```python
from build123d import *

# Parameters (mm, degrees)
BOSS_EXTRUDE2_DEPTH      = 3.5
CUT_EXTRUDE3_DEPTH       = 161.765145163
CUT_EXTRUDE3_DEPTH_BACK  = 161.765145163
SKETCH3_R                = 1.625
CUT_EXTRUDE6_DEPTH       = 161.765145163
CUT_EXTRUDE6_DEPTH_BACK  = 161.765145163
SKETCH6_R                = 15
SKETCH8_R                = 1.5
CUT_EXTRUDE7_DEPTH       = 3.5
CIRPATTERN1_COUNT        = 4
CUT_EXTRUDE12_DEPTH      = 161.765145163
CUT_EXTRUDE12_DEPTH_BACK = 161.765145163
SKETCH20_W               = 15
SKETCH20_H               = 15
FILLET2_R                = 25
FILLET3_R                = 4
SKETCH21_R               = 2.5
BOSS_EXTRUDE4_DEPTH      = 3
SKETCH22_R               = 1.6
CUT_EXTRUDE13_DEPTH      = 158.947840775
SKETCH24_R               = 2.4
BOSS_EXTRUDE6_DEPTH      = 3.5
CUT_EXTRUDE14_DEPTH      = 158.969207144
CUT_EXTRUDE14_DEPTH_BACK = 158.969207144
SKETCH25_R               = 1.6
CUT_EXTRUDE15_DEPTH      = 158.852844148
CUT_EXTRUDE15_DEPTH_BACK = 158.852844148
SKETCH26_R               = 9.404630818
CUT_EXTRUDE16_DEPTH      = 158.852844148
CUT_EXTRUDE16_DEPTH_BACK = 158.852844148
CUT_EXTRUDE17_DEPTH      = 158.969207144
CUT_EXTRUDE17_DEPTH_BACK = 158.969207144
SKETCH28_R               = 10


with BuildPart() as part:
    # Sketch1 → Boss-Extrude2 (new body)
    with BuildSketch(Plane(origin=(0, 0, 0), x_dir=(1, 0, 0), z_dir=(0, 1, 0))):
        Polygon((0, -113.651181031), (80.363520797, -80.363520797), (113.651181031, 0), (80.363520797, 80.363520797), (0, 113.651181031), (-80.363520797, 80.363520797), (-113.651181031, 0), (-80.363520797, -80.363520797), align=None)
    extrude(amount=BOSS_EXTRUDE2_DEPTH)

    # Sketch3 → Cut-Extrude3 (cut, two sides: drawn at the far end of the back side and taken through both)
    with BuildSketch(Plane(origin=(0, 3.5, 0), x_dir=(1, 0, 0), z_dir=(0, 1, 0)).offset(-CUT_EXTRUDE3_DEPTH_BACK)):
        with Locations(Location((-75, -75, 0), (0, 0, 270))):
            Circle(SKETCH3_R)
        with Locations(Location((75, -75, 0), (0, 0, 270))):
            Circle(SKETCH3_R)
        with Locations(Location((75, 75, 0), (0, 0, 270))):
            Circle(SKETCH3_R)
        with Locations(Location((-75, 75, 0), (0, 0, 270))):
            Circle(SKETCH3_R)
    extrude(amount=CUT_EXTRUDE3_DEPTH + CUT_EXTRUDE3_DEPTH_BACK, mode=Mode.SUBTRACT)

    # Sketch6 → Cut-Extrude6 (cut, two sides: drawn at the far end of the back side and taken through both)
    with BuildSketch(Plane(origin=(0, 3.5, 0), x_dir=(1, 0, 0), z_dir=(0, 1, 0)).offset(-CUT_EXTRUDE6_DEPTH_BACK)):
        with Locations(Location((0, 0, 0), (0, 0, 270))):
            Circle(SKETCH6_R)
    extrude(amount=CUT_EXTRUDE6_DEPTH + CUT_EXTRUDE6_DEPTH_BACK, mode=Mode.SUBTRACT)

    # Sketch8 → Cut-Extrude7 (cut)
    with BuildSketch(Plane(origin=(0, 3.5, 0), x_dir=(1, 0, 0), z_dir=(0, 1, 0))):
        with Locations(Location((-15, -71.401181031, 0), (0, 0, 270))):
            Circle(SKETCH8_R)
        with Locations(Location((15, -71.401181031, 0), (0, 0, 270))):
            Circle(SKETCH8_R)
        with Locations(Location((-15, -101.151181031, 0), (0, 0, 270))):
            Circle(SKETCH8_R)
        with Locations(Location((15, -101.151181031, 0), (0, 0, 270))):
            Circle(SKETCH8_R)
    cut_extrude7 = extrude(amount=-CUT_EXTRUDE7_DEPTH, mode=Mode.SUBTRACT)

    # CirPattern1: Cut-Extrude7 ×4 about axis
    cirpattern1_axis = Axis((0, 0, 0), (0, 1, 0))
    for i in range(1, CIRPATTERN1_COUNT):
        add(cut_extrude7.rotate(cirpattern1_axis, i * 360 / CIRPATTERN1_COUNT), mode=Mode.SUBTRACT)

    # Sketch20 → Cut-Extrude12 (cut, two sides: drawn at the far end of the back side and taken through both)
    with BuildSketch(Plane(origin=(0, 3.5, 0), x_dir=(1, 0, 0), z_dir=(0, 1, 0)).offset(-CUT_EXTRUDE12_DEPTH_BACK)):
        with Locations((33.5, 78.901181031)):
            Rectangle(SKETCH20_W, SKETCH20_H)
    extrude(amount=CUT_EXTRUDE12_DEPTH + CUT_EXTRUDE12_DEPTH_BACK, mode=Mode.SUBTRACT)

    # Fillet2
    fillet2_edges = [part.edges().sort_by_distance(p)[0] for p in [
        (-113.651181031, 1.75, 0),
        (0, 1.75, -113.651181031),
        (113.651181031, 1.75, 0),
        (0, 1.75, 113.651181031),
    ]]
    fillet(fillet2_edges, radius=FILLET2_R)

    # Fillet3
    fillet3_edges = [part.edges().sort_by_distance(p)[0] for p in [
        (41, 1.75, -86.401181031),
    ]]
    fillet(fillet3_edges, radius=FILLET3_R)

    # Sketch21 → Boss-Extrude4 (add)
    with BuildSketch(Plane.XZ):
        with Locations(Location((-8.867969273, 25.52523978, 0), (0, 0, 90))):
            Circle(SKETCH21_R)
        with Locations(Location((25.310885524, -8.653615016, 0), (0, 0, 90))):
            Circle(SKETCH21_R)
        with Locations(Location((44.25922594, 78.652434993, 0), (0, 0, 90))):
            Circle(SKETCH21_R)
        with Locations(Location((83.736431848, 49.771931307, 0), (0, 0, 90))):
            Circle(SKETCH21_R)
    extrude(amount=BOSS_EXTRUDE4_DEPTH)

    # Sketch22 → Cut-Extrude13 (cut, through all)
    with BuildSketch(Plane.XZ.offset(3)):
        with Locations(Location((83.736431848, 49.771931307, 0), (0, 0, 270))):
            Circle(SKETCH22_R)
        with Locations(Location((25.310885524, -8.653615016, 0), (0, 0, 270))):
            Circle(SKETCH22_R)
        with Locations(Location((-8.867969273, 25.52523978, 0), (0, 0, 270))):
            Circle(SKETCH22_R)
        with Locations(Location((44.25922594, 78.652434993, 0), (0, 0, 270))):
            Circle(SKETCH22_R)
    extrude(amount=-CUT_EXTRUDE13_DEPTH, mode=Mode.SUBTRACT)

    # Sketch24 → Boss-Extrude6 (add)
    with BuildSketch(Plane.XZ):
        with Locations(Location((-64.472580457, -31.0267951, 0), (0, 0, 90))):
            Circle(SKETCH24_R)
        with Locations(Location((-29.019501349, -37.278129496, 0), (0, 0, 90))):
            Circle(SKETCH24_R)
        with Locations(Location((-35.270835745, -72.731208605, 0), (0, 0, 90))):
            Circle(SKETCH24_R)
        with Locations(Location((-70.723914853, -66.479874209, 0), (0, 0, 90))):
            Circle(SKETCH24_R)
    extrude(amount=BOSS_EXTRUDE6_DEPTH)

    # Sketch25 → Cut-Extrude14 (cut, two sides: drawn at the far end of the back side and taken through both)
    with BuildSketch(Plane.XZ.offset(3.5).offset(-CUT_EXTRUDE14_DEPTH_BACK)):
        with Locations(Location((-29.019501349, -37.278129496, 0), (0, 0, 270))):
            Circle(SKETCH25_R)
        with Locations(Location((-64.472580457, -31.0267951, 0), (0, 0, 270))):
            Circle(SKETCH25_R)
        with Locations(Location((-70.723914853, -66.479874209, 0), (0, 0, 270))):
            Circle(SKETCH25_R)
        with Locations(Location((-35.270835745, -72.731208605, 0), (0, 0, 270))):
            Circle(SKETCH25_R)
    extrude(amount=CUT_EXTRUDE14_DEPTH + CUT_EXTRUDE14_DEPTH_BACK, mode=Mode.SUBTRACT)

    # Sketch26 → Cut-Extrude15 (cut, two sides: drawn at the far end of the back side and taken through both)
    with BuildSketch(Plane.XZ.offset(-CUT_EXTRUDE15_DEPTH_BACK)):
        with Locations(Location((-60.741403737, 60.741403737, 0), (0, 0, 270))):
            Circle(SKETCH26_R)
        with Locations(Location((60.741403737, -60.741403737, 0), (0, 0, 270))):
            Circle(SKETCH26_R)
    extrude(amount=CUT_EXTRUDE15_DEPTH + CUT_EXTRUDE15_DEPTH_BACK, mode=Mode.SUBTRACT)

    # Sketch27 → Cut-Extrude16 (cut, two sides: drawn at the far end of the back side and taken through both)
    with BuildSketch(Plane.XZ.offset(-CUT_EXTRUDE16_DEPTH_BACK)):
        Polygon((7.39951467, 57.553878611), (11.642155357, 53.311237924), (-9.571048078, 32.098034488), (-13.813688765, 36.340675176), align=None)
        Polygon((32.098034488, -9.571048078), (36.340675176, -13.813688765), (57.553878611, 7.39951467), (53.311237924, 11.642155357), align=None)
    extrude(amount=CUT_EXTRUDE16_DEPTH + CUT_EXTRUDE16_DEPTH_BACK, mode=Mode.SUBTRACT)

    # Sketch28 → Cut-Extrude17 (cut, two sides: drawn at the far end of the back side and taken through both)
    with BuildSketch(Plane(origin=(0, 3.5, 0), x_dir=(1, 0, 0), z_dir=(0, 1, 0)).offset(-CUT_EXTRUDE17_DEPTH_BACK)):
        with Locations(Location((-34.694923367, -27.917780902, 0), (0, 0, 270))):
            Circle(SKETCH28_R)
    extrude(amount=CUT_EXTRUDE17_DEPTH + CUT_EXTRUDE17_DEPTH_BACK, mode=Mode.SUBTRACT)


solid = part.part
```
CAD build for the part. Positions are in the model's coordinates, mm. A direction names the side the tool comes from. Round coordinates to 2 decimals unless told otherwise and drop trailing zeros. Write each loop counter-clockwise with the first axis right and the second up, starting at its lowest first coordinate (ties: lowest second). Pieces come first, ordered by that corner, then holes. Notation, with made-up numbers: (3.5, -10) - (18.5, -10) arc R20 cw to (18.5, 23) - close; hole circle Ø1 at (34.25, 46.25). An arc over 180 degrees is marked (long way). Return JSON: item names as keys, results as strings. Group by question number.
Item 1: Flat gauge pins, fed straight in: pin 1 Ø3 at (y, z) = (1.5, -82.5) entering from +X; pin 2 Ø1 at (y, z) = (0.5, 40) entering from -X; pin 3 Ø2 at (y, z) = (0.5, 43) entering from -X; pin 4 Ø2.5 at (x, z) = (-101.15, -15) entering from -Y. Where does each tip first touch, or does it go through?
Item 2: Band-saw the part on D-D on z = -89. List the corners of the cut face in (x, y), plus the area to 3 significant figures.
Item 3: Mould opens along Z. For faces 1 (the face through (-45.46, 1.73, 94.82)), 2 (the face through (-3.356, 1.774, 46.799)), 3 (the face through (-10.558, -1.479, 23.683)) say: +Z half, -Z half, draft (parallel to the pull), parting line (faces both ways), or undercut.
Item 4: Band-saw the part on A-A on z = 60.5. List the corners of the cut face in (x, y).
Item 5: Band-saw the part on C-C on z = -48. List the corners of the cut face in (x, y), plus the area to 3 significant figures.
Item 6: Band-saw the part on B-B on x = -55.5. List the corners of the cut face in (y, z).
Item 7: 3-axis set-ups, long thin cutter, end or side, ignore diameter. For faces 4 (the face through (-33.142, -1.726, -71.624)), 5 (the face through (46.799, 1.774, -3.356)), 6 (the face through (95.23, 1.73, -44.47)): which of +Z, -Z, +X, -X, +Y, -Y reach the whole face in a straight line?
Item 8: Probe probe 1 along Z at (x, y) = (75, 1.25) (3 decimals); probe 2 along X at (y, z) = (1.75, 0). List the from-to ranges inside material, lowest first.
Resolved:
{
 "1": {"pin 1": "stops at x = 78.83", "pin 2": "stops at x = -97.29", "pin 3": "stops at x = -96.25", "pin 4": "passes through"},
 "2": {"outline": "(-59.51, 0) - (59.51, 0) - (59.51, 3.5) - (-59.51, 3.5) - close", "area": "417 mm²"},
 "3": {"face 1": "+Z half", "face 2": "undercut", "face 3": "parting line"},
 "4": {"outline": "(-88.59, 0) - (-70.14, 0) - (-70.14, 3.5) - (-88.59, 3.5) - close; (-51.34, 0) - (88.59, 0) - (88.59, 3.5) - (-51.34, 3.5) - close"},
 "5": {"outline": "(-93.77, 0) - (93.77, 0) - (93.77, 3.5) - (-93.77, 3.5) - close", "area": "656 mm²"},
 "6": {"outline": "(0, -90.66) - (3.5, -90.66) - (3.5, 52.93) - (0, 52.93) - close; (0, 68.55) - (3.5, 68.55) - (3.5, 90.66) - (0, 90.66) - close"},
 "7": {"face 4": "-Y", "face 5": "+Y, -Y", "face 6": "-Z, +X, +Y, -Y"},
 "8": {"probe 1": "z = -82.585 to -76.625, -73.375 to 73.375, 76.625 to 82.585", "probe 2": "x = -111.59 to -15, 15 to 41.67, 50.15 to 111.59"}
}
